Source: CAD feature listing. Evaluate the final solid. Frame: model axes, mm. Face numbers are marked on the shaded views. Give positions to 0.01 mm unless a question says otherwise; leave off trailing zeros. Loops run counter-clockwise (first coordinate to the right, second up) from the corner with the lowest first, then second, coordinate; pieces in that order, holes last.
```python
from build123d import *

# Parameters (mm, degrees)
IZIM1_W                              = 100
IZIM1_H                              = 56
IZIM1_R                              = 9.5
IZIM1_R_2                            = 2.031053151
Y_KSEKLIK_EKSTR_ZYON1_DEPTH          = 8
IZIM2_R                              = 11
KES_EKSTR_ZYON1_DEPTH                = 10
IZIM3_R                              = 1.25
KES_EKSTR_ZYON2_DEPTH                = 10
M5_HELISARMAL_I_IN_Z_VANA_MATKAB_1_D = 5.2


with BuildPart() as part:
    # Çizim1 → Yükseklik-Ekstrüzyon1 (new body)
    with BuildSketch(Plane.XY):
        with Locations((-2.031053151, 0.257686676)):
            Rectangle(IZIM1_W, IZIM1_H)
        with Locations((-32.031053151, 3.257686676)):
            Circle(IZIM1_R, mode=Mode.SUBTRACT)
        with Locations((27.968946849, 3.257686676)):
            Circle(IZIM1_R, mode=Mode.SUBTRACT)
        with Locations((-2.031053151, 3.257686676)):
            Circle(IZIM1_R_2, mode=Mode.SUBTRACT)
    extrude(amount=Y_KSEKLIK_EKSTR_ZYON1_DEPTH)

    # Çizim2 → Kes-Ekstrüzyon1 (cut)
    with BuildSketch(Plane.XY.offset(8)):
        with Locations((-2.031053151, 3.257686676)):
            Circle(IZIM2_R)
    extrude(amount=-KES_EKSTR_ZYON1_DEPTH, mode=Mode.SUBTRACT)

    # Çizim3 → Kes-Ekstrüzyon2 (cut)
    with BuildSketch(Plane(origin=(0, 0, 0), x_dir=(-1, 0, 0), z_dir=(0, 0, -1))):
        with Locations((-13.468946849, 19.617369517)):
            Circle(IZIM3_R)
        with Locations((17.531053151, 18.757686676)):
            Circle(IZIM3_R)
        with Locations((16.962368033, -12.242313324)):
            Circle(IZIM3_R)
        with Locations((-14.037631967, -11.382630483)):
            Circle(IZIM3_R)
    extrude(amount=-KES_EKSTR_ZYON2_DEPTH, mode=Mode.SUBTRACT)

    # M5 Helisarmal için Zıvana matkabı1 (through all)
    with Locations(Plane(origin=(-42.031053151, 20.757686676, 8), x_dir=(1, 0, 0), z_dir=(0, 0, 1))):
        with Locations((0, 0), (80, 0), (80, -33), (0, -33)):
            Hole(M5_HELISARMAL_I_IN_Z_VANA_MATKAB_1_D / 2)


solid = part.part
```
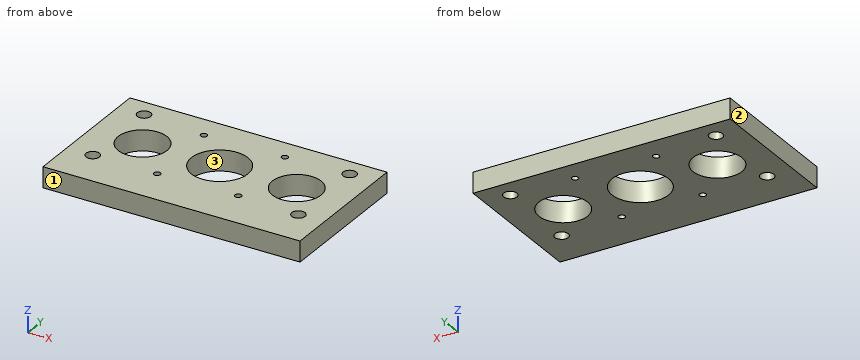
(1) Section C-C, the plane x = -36. Return the cut outline in (y, z), then the cut area to 3 significant figures.
A:
outline: (-27.74, 0) - (-5.37, 0) - (-5.37, 8) - (-27.74, 8) - close; (11.89, 0) - (28.26, 0) - (28.26, 8) - (11.89, 8) - close
area: 310 mm2
(2) Mould query, pull axis X, two halves, no side actions, for the marked faces 1, 2 and 3. Classes: pulls with the +X half, pulls with the -X half, needs draft (parallel to the pull), parting line crosses it, or undercut.
A:
face 1: needs draft
face 2: pulls with the -X half
face 3: undercut
(3) First-contact query: pin 1 (5 mm diameter, centred on x = -9.5, y = 12.5, fed in from -Z); pin 2 (3 mm diameter, centred on x = 37.97, y = -12.24, fed in from +Z). Flat tips, straight axial feed; report the tip coordinate or a pass-through.
A:
pin 1: stops at z = 0
pin 2: passes through
(4) Section B-B, the plane z = 1.5. Count the separate pieces of the cut face and the enclosed holes in it, then the cut area to 3 significant figures.
A:
separate pieces: 1
enclosed holes: 11
area: 4,550 mm2
(5) Section A-A, the plane x = 25.5. Return the cut outline in (y, z).
A:
outline: (-27.74, 0) - (-5.92, 0) - (-5.92, 8) - (-27.74, 8) - close; (12.43, 0) - (28.26, 0) - (28.26, 8) - (12.43, 8) - close
(6) Ray query, line 1 along X through (y, z) = (3, 4.25); line 2 along Y through (x, z) = (38, 5.5); line 3 along Y through (x, z) = (36.5, 3.5). Return the intervals inside material, ascending.
A:
line 1: x = -52.03 to -41.53, -22.53 to -13.03, 8.97 to 18.47, 37.47 to 47.97
line 2: y = -27.74 to -14.84, -9.64 to 18.16, 23.36 to 28.26
line 3: y = -27.74 to -14.39, -10.1 to -0.92, 7.44 to 18.61, 22.9 to 28.26
